CAD build for the part. Positions are in the model's coordinates, mm. Face numbers are marked on the shaded views. A direction names the side the tool comes from. Give positions to 0.01 mm unless a question says otherwise; leave off trailing zeros. Loops run counter-clockwise (first coordinate to the right, second up) from the corner with the lowest first, then second, coordinate; pieces in that order, holes last. Notation, with made-up numbers: M -22.5,-10 L -4.5,-10 A24 ccw -4.5,26 Z; hole C -38.5,34.5 d9. An arc over 180 degrees is marked long. One line per question, with ' | ' between items.
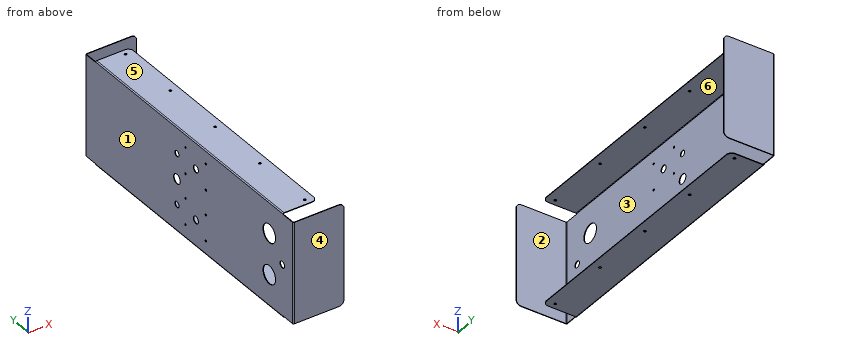
```python
from build123d import *

# Parameters (mm, degrees)
BASE_FLANGE1_DEPTH           = 147.5
EDGE_FLANGE1_DEPTH           = 792
EDGE_FLANGE1_BEND_DEPTH      = 792
F_7_0_7_DIAMETER_HOLE1_D     = 7
F_7_0_7_DIAMETER_HOLE1_DEPTH = 1.5
FILLET1_R                    = 15
SKETCH14_R                   = 26.5
CUT_EXTRUDE1_DEPTH           = 488.566918484
M16_CLEARANCE_HOLE1_D        = 19
M5_CLEARANCE_HOLE1_D         = 5.8
M20_CLEARANCE_HOLE1_D        = 21
CUT_EXTRUDE2_DEPTH           = 488.566918484
CUT_EXTRUDE3_DEPTH           = 488.566918484


# Sheet-metal steps are written as plain solids
with BuildPart() as part:
    # Sketch1 → Base-Flange1 (new, symmetric)
    with BuildSketch(Plane.XY):
        with BuildLine():
            Line((147, 438), (1.5, 438))
            ThreePointArc((1.5, 438), (0.439339828, 437.560660172), (0, 436.5))
            Line((0, 436.5), (0, -436.5))
            ThreePointArc((0, -436.5), (0.439339828, -437.560660172), (1.5, -438))
            Line((1.5, -438), (147, -438))
            Line((147, -438), (147, -439.5))
            Line((147, -439.5), (1.5, -439.5))
            ThreePointArc((1.5, -439.5), (-0.621320344, -438.621320344), (-1.5, -436.5))
            Line((-1.5, -436.5), (-1.5, 436.5))
            ThreePointArc((-1.5, 436.5), (-0.621320344, 438.621320344), (1.5, 439.5))
            Line((1.5, 439.5), (147, 439.5))
            Line((147, 439.5), (147, 438))
        make_face()
    extrude(amount=BASE_FLANGE1_DEPTH, both=True)

    # Edge-Flange1 section (across the edge) → Edge-Flange1 (add)
    with BuildSketch(Plane(origin=(0, 396, 150), x_dir=(0, 0, -1), z_dir=(0, -1, 0))):
        with BuildLine():
            Line((-1.5, 1.5), (-1.5, 98.5))
            Line((-1.5, 98.5), (0, 98.5))
            Line((0, 98.5), (0, 1.5))
            ThreePointArc((0, 1.5), (0.439339828, 0.439339828), (1.5, 0))
            Line((1.5, 0), (2.5, 0))
            Line((2.5, 0), (2.5, -1.5))
            Line((2.5, -1.5), (1.5, -1.5))
            ThreePointArc((1.5, -1.5), (-0.621320344, -0.621320344), (-1.5, 1.5))
        make_face()
    extrude(amount=EDGE_FLANGE1_DEPTH)

    # Edge-Flange1 section 2 (across the edge) → Edge-Flange1 bend (add)
    with BuildSketch(Plane(origin=(0, -396, -150), x_dir=(0, 0, 1), z_dir=(0, 1, 0))):
        with BuildLine():
            Line((-1.5, 1.5), (-1.5, 98.5))
            Line((-1.5, 98.5), (0, 98.5))
            Line((0, 98.5), (0, 1.5))
            ThreePointArc((0, 1.5), (0.439339828, 0.439339828), (1.5, 0))
            Line((1.5, 0), (2.5, 0))
            Line((2.5, 0), (2.5, -1.5))
            Line((2.5, -1.5), (1.5, -1.5))
            ThreePointArc((1.5, -1.5), (-0.621320344, -0.621320344), (-1.5, 1.5))
        make_face()
    extrude(amount=EDGE_FLANGE1_BEND_DEPTH)

    # Ø7.0 (7) Diameter Hole1
    with Locations(Plane(origin=(0, 0, 150), x_dir=(-1, 0, 0), z_dir=(0, 0, -1))):
        with Locations((-74.25, 379.5), (-74.25, 190), (-74.25, 0.5), (-74.25, -189), (-74.25, -378.5)):
            f_7_0_7_diameter_hole1 = Hole(F_7_0_7_DIAMETER_HOLE1_D / 2, depth=F_7_0_7_DIAMETER_HOLE1_DEPTH)

    # Mirror1: Ø7.0 (7) Diameter Hole1 across plane
    add(f_7_0_7_diameter_hole1.mirror(Plane.XY), mode=Mode.SUBTRACT)

    # Fillet1
    fillet1_edges = [part.edges().sort_by_distance(p)[0] for p in [
        (147, 438.75, -147.5),
        (147, -438.75, -147.5),
        (147, 438.75, 147.5),
        (98.5, 396, 150.75),
        (98.5, -396, 150.75),
        (98.5, -396, -150.75),
        (98.5, 396, -150.75),
        (147, -438.75, 147.5),
    ]]
    fillet(fillet1_edges, radius=FILLET1_R)

    # Sketch14 → Cut-Extrude1 (cut, through all)
    with BuildSketch(Plane(origin=(0, 0, 0), x_dir=(0, 0, -1), z_dir=(1, 0, 0))):
        with Locations((-60, -338)):
            Circle(SKETCH14_R)
        with Locations((60, -338)):
            Circle(SKETCH14_R)
    extrude(amount=-CUT_EXTRUDE1_DEPTH, mode=Mode.SUBTRACT)

    # M16 Clearance Hole1 (through all)
    with Locations(Plane(origin=(0, 0, 0), x_dir=(0, 0, -1), z_dir=(1, 0, 0))):
        with Locations((0, -393)):
            Hole(M16_CLEARANCE_HOLE1_D / 2)

    # M5 Clearance Hole1 (through all)
    with Locations(Plane(origin=(0, 0, 0), x_dir=(0, 0, -1), z_dir=(1, 0, 0))):
        with Locations((-112, 16.324175824), (-36, -69.675824176), (-112, -69.675824176), (-36, 16.324175824)):
            m5_clearance_hole1 = Hole(M5_CLEARANCE_HOLE1_D / 2)

    # Mirror2: M5 Clearance Hole1 across plane
    add(m5_clearance_hole1.mirror(Plane.XY), mode=Mode.SUBTRACT)

    # M20 Clearance Hole1 (through all)
    with Locations(Plane(origin=(0, 0, 0), x_dir=(0, 0, -1), z_dir=(1, 0, 0))):
        with Locations((-74, -27.5), (74, -27.5)):
            Hole(M20_CLEARANCE_HOLE1_D / 2)

    # Sketch22 → Cut-Extrude2 (cut, through all)
    with BuildSketch(Plane(origin=(0, 0, 0), x_dir=(0, 0, -1), z_dir=(1, 0, 0))):
        with BuildLine():
            Line((-82, 49.627718677), (-82, 55.372281323))
            ThreePointArc((-82, 55.372281323), (-74, 61), (-66, 55.372281323))
            Line((-66, 55.372281323), (-66, 49.627718677))
            ThreePointArc((-66, 49.627718677), (-74, 44), (-82, 49.627718677))
        make_face()
    cut_extrude2 = extrude(amount=-CUT_EXTRUDE2_DEPTH, mode=Mode.SUBTRACT)

    # Mirror3: Cut-Extrude2 across plane
    add(cut_extrude2.mirror(Plane.XY), mode=Mode.SUBTRACT)

    # Sketch23 → Cut-Extrude3 (cut, through all)
    with BuildSketch(Plane(origin=(0, 0, 0), x_dir=(0, 0, -1), z_dir=(1, 0, 0))):
        with BuildLine():
            Line((-1.65, 67.5), (-1.65, 66.402427846))
            ThreePointArc((-1.65, 66.402427846), (0, 38.5), (1.65, 66.402427846))
            Line((1.65, 66.402427846), (1.65, 67.5))
            Line((1.65, 67.5), (-1.65, 67.5))
        make_face()
    extrude(amount=-CUT_EXTRUDE3_DEPTH, mode=Mode.SUBTRACT)


solid = part.part
```
Item 1: Saw through at B-B on z = 74. Give the cut face in (x, y).
Conclusion:
outline: M -1.5,-436.5 A3 ccw 1.5,-439.5 L 147,-439.5 L 147,-438 L 1.5,-438 A1.5 cw 0,-436.5 L 0,-360.5 L -1.5,-360.5 Z; M -1.5,-315.5 L 0,-315.5 L 0,-38 L -1.5,-38 Z; M -1.5,-17 L 0,-17 L 0,44 L -1.5,44 Z; M -1.5,61 L 0,61 L 0,436.5 A1.5 cw 1.5,438 L 147,438 L 147,439.5 L 1.5,439.5 A3 ccw -1.5,436.5 Z
Item 2: Drop flat-ended pins along their axis: P1, Ø0.5, axis at x = -0.5, y = 67, coming from the +Z side; P2, Ø1.2, axis at x = -0.5, y = 53, coming from the -Z side; P3, Ø12, axis at y = -120.5, z = 78.5, coming from the +X side. Give the stop position or say it passes through.
Conclusion:
P1: z = 150.94 | P2: z = -151.15 | P3: x = 0
Item 3: Drill centre lines: line 1 along Y through (x, z) = (74.25, 151); line 2 along Y through (x, z) = (-1.1, 112); line 3 along Y through (x, z) = (41.5, -114.5). Where is each one in solid material? Low to high. Write a range as [from, to].
Conclusion:
line 1: [-396, -382], [-375, -192.5], [-185.5, -3], [4, 186.5], [193.5, 376], [383, 396] | line 2: [-438, -72.58], [-66.78, 13.42], [19.22, 438] | line 3: [-439.5, -438], [438, 439.5]
Item 4: Saw through at A-A on x = 29. Give the cut face in (y, z).
Conclusion:
outline: M -439.5,-147.5 L -438,-147.5 L -438,147.5 L -439.5,147.5 Z; M -396,-151.5 L 396,-151.5 L 396,-150 L -396,-150 Z; M -396,150 L 396,150 L 396,151.5 L -396,151.5 Z; M 438,-147.5 L 439.5,-147.5 L 439.5,147.5 L 438,147.5 Z
Item 5: Saw through at C-C on y = -158. Give the cut face in (x, z).
Conclusion:
outline: M -1.5,-148.5 A3 ccw 1.5,-151.5 L 98.5,-151.5 L 98.5,-150 L 1.5,-150 A1.5 cw 0,-148.5 L 0,148.5 A1.5 cw 1.5,150 L 98.5,150 L 98.5,151.5 L 1.5,151.5 A3 ccw -1.5,148.5 Z
Item 6: 3-axis set-ups, long thin cutter, end or side, ignore diameter. For the marked faces 1 and 2: which of +Z, -Z, +X, -X, +Y, -Y reach the whole face in a straight line?
Conclusion:
face 1: +Z, -Z, -X, +Y, -Y | face 2: +Z, -Z, +X
Item 7: Mould opens along Z. For the marked faces 3, 4, 5 and 6 say: pulls with the +Z half, pulls with the -Z half, needs draft (parallel to the pull), parting line crosses it, or undercut.
Conclusion:
face 3: undercut | face 4: needs draft | face 5: pulls with the +Z half | face 6: undercut
